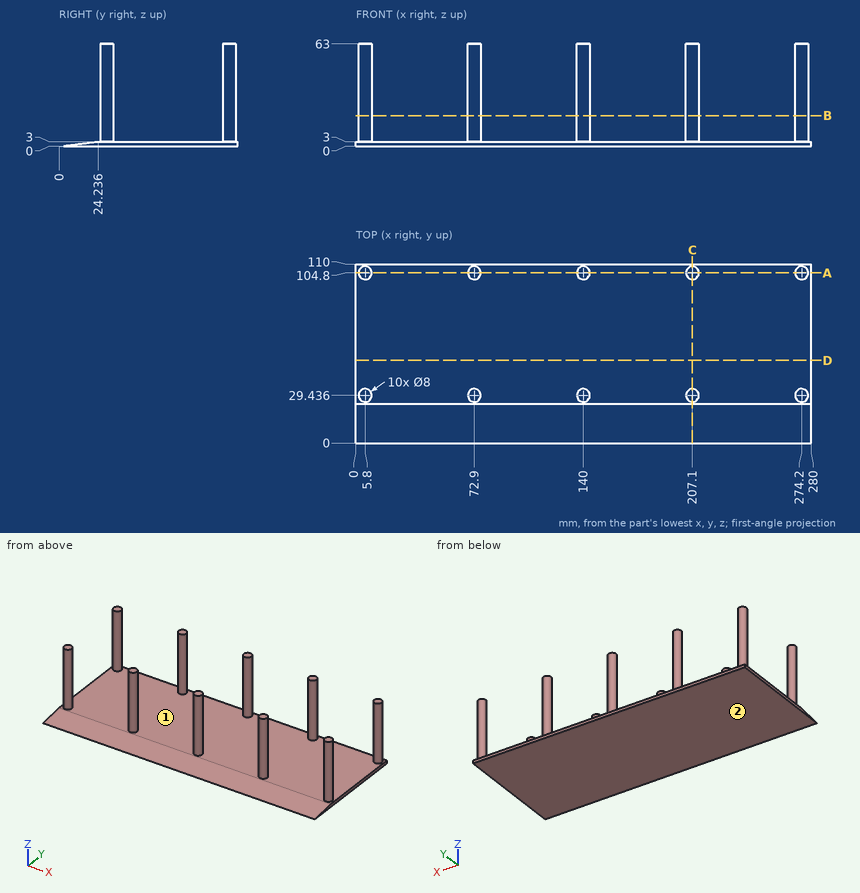
Design review of the part shown in the three views and the two pictorial views. Dimensions are in mm from the part's minimum x, y and z. Coordinates: 2 decimals unless noted, no trailing zeros. Write each loop counter-clockwise with the first axis right and the second up, starting at its lowest first coordinate (ties: lowest second). Pieces come first, ordered by that corner, then holes.
1) We need section B-B on z = 19. Count the separate pieces of the cut face and the enclosed holes in it, then the cut area to 3 significant figures.
2) We need section C-C on x = 207.1. State the section outline as (y, z) points, then the cut area to 3 significant figures.
3) To check wall thickness, follow probe 1 along X at (y, z) = (30, 36); probe 2 along Z at (x, y) = (86.5, 39); probe 3 along Y at (x, z) = (74, 53). State the ranges of each line that lie inside material, in increasing order.
4) We need section A-A on y = 104.8. State the section outline as (x, z) points.
5) The part is to be moulded in two halves that separate along X. For the marked faces 1 and 2, say which applies: pulls with the +X half, pulls with the -X half, needs draft (parallel to the pull), parting line crosses it, or undercut.
6) We need section D-D on y = 51. State the section outline as (x, z) points.
Answer list:
1. separate pieces: 10
1. enclosed holes: 0
1. area: 503 mm2
2. outline: (0, 0) - (110, 0) - (110, 3) - (108.8, 3) - (108.8, 63) - (100.8, 63) - (100.8, 3) - (33.44, 3) - (33.44, 63) - (25.44, 63) - (25.44, 3) - (24.24, 3) - close
2. area: 1,250 mm2
3. probe 1: x = 1.84 to 9.76, 68.94 to 76.86, 136.04 to 143.96, 203.14 to 211.06, 270.24 to 278.16
3. probe 2: z = 0 to 3
3. probe 3: y = 25.59 to 33.28, 100.95 to 108.65
4. outline: (0, 0) - (280, 0) - (280, 3) - (278.2, 3) - (278.2, 63) - (270.2, 63) - (270.2, 3) - (211.1, 3) - (211.1, 63) - (203.1, 63) - (203.1, 3) - (144, 3) - (144, 63) - (136, 63) - (136, 3) - (76.9, 3) - (76.9, 63) - (68.9, 63) - (68.9, 3) - (9.8, 3) - (9.8, 63) - (1.8, 63) - (1.8, 3) - (0, 3) - close
5. face 1: undercut
5. face 2: needs draft
6. outline: (0, 0) - (280, 0) - (280, 3) - (0, 3) - close
